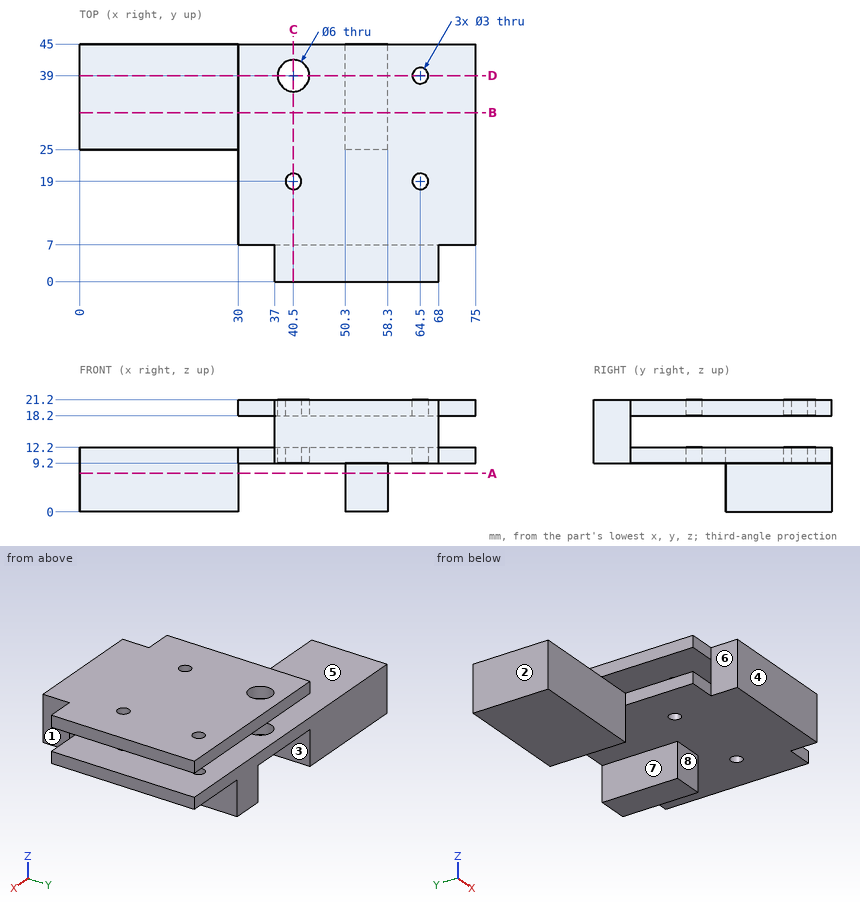
Could you check a few things on this drawing? It's one solid part, dimensions in mm from its lowest x, y, z. A direction names the side the tool comes from. Coordinates: 2 decimals unless noted, no trailing zeros. Write each loop counter-clockwise with the first axis right and the second up, starting at its lowest first coordinate (ties: lowest second). Pieces come first, ordered by that corner, then holes. Notation, with made-up numbers: M 22.5,53 L 31.5,53 A21 ccw 31.5,75 Z; hole C 56,11.5 d9. An arc over 180 degrees is marked long. Answer as CSV lines item,"result". Start each with the question number.
Q1. Suppose I cut it at D-D, the plane y = 39. State how many separate pieces and enclosed holes the cut face has, then the cut area to 3 significant figures.
Q2. Will these pins go through, and if not, where does the flat tip stop? pin 1 Ø3.5 at (y, z) = (5, 15) entering from -X; pin 2 Ø1.5 at (x, z) = (71, 19.5) entering from -Y; pin 3 Ø4 at (x, z) = (54.5, 4) entering from -Y.
Q3. If we mould it in two halves opening along X, with no side actions, what happens to the marked faces 1, 2, 3 and 4? For each: pulls with the +X half, pulls with the -X half, needs draft (parallel to the pull), parting line crosses it, or undercut.
Q4. Suppose I cut it at C-C, the plane x = 40.5. List the corners of the cut face in (y, z) for me.
Q5. Suppose I cut it at B-B, the plane y = 32. List the corners of the cut face in (x, z) for me, then the cut area to 3 significant figures.
Q6. I need wall thicknesses on probe 1 along Y at (x, z) = (40.5, 11.35); probe 2 along Y at (x, z) = (64.5, 11.4); probe 3 along Z at (x, y) = (58, 24.5). Which ranges of each line are inside material? Lowest first, please. Write a range as [from, to].
Q7. For the marked faces 5, 6, 7 and 8, which set-ups out of +Z, -Z, +X, -X, +Y, -Y let a thin tool reach every point of the face, with its end or its side?
Q8. Suppose I cut it at A-A, the plane z = 7.25. List the corners of the cut face in (x, y) for me.
Entries:
1,separate pieces,"6"
1,enclosed holes,"0"
1,area,"656 mm²"
2,pin 1,"stops at x = 37"
2,pin 2,"stops at y = 7"
2,pin 3,"stops at y = 25"
3,face 1,"pulls with the +X half"
3,face 2,"pulls with the -X half"
3,face 3,"undercut"
3,face 4,"needs draft"
4,outline,"M 0,9.2 L 17.5,9.2 L 17.5,12.2 L 7,12.2 L 7,18.2 L 17.5,18.2 L 17.5,21.2 L 0,21.2 Z; M 20.5,9.2 L 36,9.2 L 36,12.2 L 20.5,12.2 Z; M 20.5,18.2 L 36,18.2 L 36,21.2 L 20.5,21.2 Z; M 42,9.2 L 45,9.2 L 45,12.2 L 42,12.2 Z; M 42,18.2 L 45,18.2 L 45,21.2 L 42,21.2 Z"
5,outline,"M 0,0 L 30,0 L 30,9.2 L 50.3,9.2 L 50.3,0 L 58.3,0 L 58.3,9.2 L 75,9.2 L 75,12.2 L 0,12.2 Z; M 30,18.2 L 75,18.2 L 75,21.2 L 30,21.2 Z"
5,area,"710 mm²"
6,probe 1,"y = [0, 17.5], [20.5, 36], [42, 45]"
6,probe 2,"y = [0, 17.5], [20.5, 37.5], [40.5, 45]"
6,probe 3,"z = [9.2, 12.2], [18.2, 21.2]"
7,face 5,"+X, -X, +Y"
7,face 6,"+Z, -Z, -X, -Y"
7,face 7,"-Z, +Y, -Y"
7,face 8,"-Z, +X, -X, -Y"
8,outline,"M 0,25 L 30,25 L 30,45 L 0,45 Z; M 50.3,25 L 58.3,25 L 58.3,45 L 50.3,45 Z"
